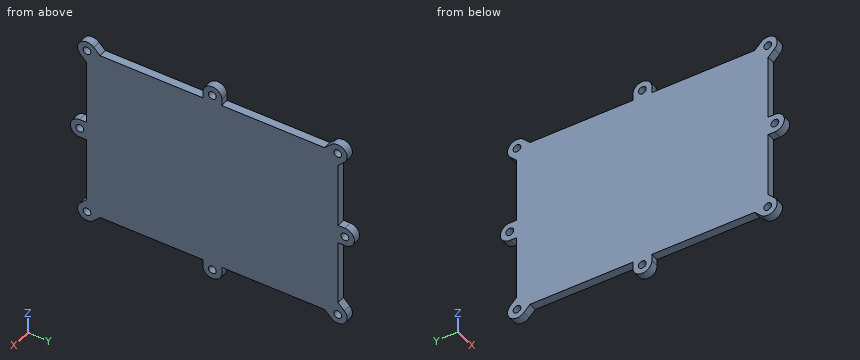
from build123d import *

# Parameters (mm, degrees)
BOSS_EXTRUDE1_DEPTH  = 4.7625
M4_CLEARANCE_HOLE1_D = 4.5


with BuildPart() as part:
    # Sketch1 → Boss-Extrude1 (new body)
    with BuildSketch(Plane(origin=(0, 0, 0), x_dir=(0, 0, -1), z_dir=(1, 0, 0))):
        with BuildLine():
            Line((-12.938571051, 72.8815), (-50.697896458, 72.8815))
            Line((-50.697896458, 72.8815), (-50.697896458, 76.7912))
            ThreePointArc((-50.697896458, 76.7912), (-56.197896458, 82.2912), (-61.697896458, 76.7912))
            Line((-61.697896458, 76.7912), (-61.697896458, 72.8815))
            Line((-61.697896458, 72.8815), (-99.457221865, 72.8815))
            Line((-99.457221865, 72.8815), (-103.084126021, 76.508404156))
            ThreePointArc((-103.084126021, 76.508404156), (-110.862300614, 76.508404156), (-110.862300614, 68.730229563))
            Line((-110.862300614, 68.730229563), (-107.235396458, 65.103325407))
            Line((-107.235396458, 65.103325407), (-107.235396458, 5.5))
            Line((-107.235396458, 5.5), (-111.145096458, 5.5))
            ThreePointArc((-111.145096458, 5.5), (-116.645096458, 0), (-111.145096458, -5.5))
            Line((-111.145096458, -5.5), (-107.235396458, -5.5))
            Line((-107.235396458, -5.5), (-107.235396458, -65.103325407))
            Line((-107.235396458, -65.103325407), (-110.862300614, -68.730229563))
            ThreePointArc((-110.862300614, -68.730229563), (-110.862300614, -76.508404156), (-103.084126021, -76.508404156))
            Line((-103.084126021, -76.508404156), (-99.457221865, -72.8815))
            Line((-99.457221865, -72.8815), (-61.697896458, -72.8815))
            Line((-61.697896458, -72.8815), (-61.697896458, -76.7912))
            ThreePointArc((-61.697896458, -76.7912), (-56.197896458, -82.2912), (-50.697896458, -76.7912))
            Line((-50.697896458, -76.7912), (-50.697896458, -72.8815))
            Line((-50.697896458, -72.8815), (-12.938571051, -72.8815))
            Line((-12.938571051, -72.8815), (-9.311666896, -76.508404156))
            ThreePointArc((-9.311666896, -76.508404156), (-1.533492302, -76.508404156), (-1.533492302, -68.730229563))
            Line((-1.533492302, -68.730229563), (-5.160396458, -65.103325407))
            Line((-5.160396458, -65.103325407), (-5.160396458, -5.5))
            Line((-5.160396458, -5.5), (-1.250696458, -5.5))
            ThreePointArc((-1.250696458, -5.5), (4.249303542, 0), (-1.250696458, 5.5))
            Line((-1.250696458, 5.5), (-5.160396458, 5.5))
            Line((-5.160396458, 5.5), (-5.160396458, 65.103325407))
            Line((-5.160396458, 65.103325407), (-1.533492302, 68.730229563))
            ThreePointArc((-1.533492302, 68.730229563), (-1.533492302, 76.508404156), (-9.311666896, 76.508404156))
            Line((-9.311666896, 76.508404156), (-12.938571051, 72.8815))
        make_face()
    extrude(amount=-BOSS_EXTRUDE1_DEPTH)

    # M4 Clearance Hole1 (through all)
    with Locations(Plane.ZY.offset(4.7625)):
        with Locations((5.422579599, -72.619316859), (1.250696458, 0), (5.422579599, 72.619316859), (106.973213317, 72.619316859), (111.145096458, 0), (106.973213317, -72.619316859), (56.197896458, -76.7912), (56.197896458, 76.7912)):
            Hole(M4_CLEARANCE_HOLE1_D / 2)


solid = part.part
Geometry: final body of the model. Coordinates: model frame, mm. Give positions to 0.01 mm unless a question says otherwise; leave off trailing zeros. Loops run counter-clockwise (first coordinate to the right, second up) from the corner with the lowest first, then second, coordinate; pieces in that order, holes last. Notation, with made-up numbers: M -23,6.5 L 5,6.5 A10 cw 5,21.5 Z; hole C 18,-24.75 d1. An arc over 180 degrees is marked long. Put each result on its own line as item: value.
1) Cut plane A-A, the plane y = 0. Return the cut outline in (x, z), plus the area to 3 significant figures.
Computed values:
outline: M -4.76,-4.25 L 0,-4.25 L 0,-1 L -4.76,-1 Z; M -4.76,3.5 L 0,3.5 L 0,108.9 L -4.76,108.9 Z; M -4.76,113.4 L 0,113.4 L 0,116.65 L -4.76,116.65 Z
area: 533 mm^2
2) Cut plane C-C, the plane z = 43.5. Return the cut outline in (x, y).
Computed values:
outline: M -4.76,-72.88 L 0,-72.88 L 0,72.88 L -4.76,72.88 Z
3) Material intervals for L1, parallel to Y at x = -0.2, z = 107.5; L2, parallel to Z at x = -0.55, y = 75; L3, parallel to Z at x = -1.55, y = -1.5, sorted ascending. Write a range as from..to.
Computed values:
L1: y = -78.09..-74.81, -70.43..-65.37, -5.5..5.5, 65.37..70.43, 74.81..78.09
L2: z = 0.46..10.82, 50.7..54.84, 57.56..61.7, 101.58..111.93
L3: z = -4.04..-0.43, 2.93..109.47, 112.82..116.44
4) First-contact query: P1, Ø2.5, axis at x = -3.5, z = 39, coming from the +Y side; P2, Ø7, axis at y = 72.62, z = 5.42, coming from the +X side; P3, Ø1.2, axis at x = -2, y = -74.5, coming from the +Z side; P4, Ø1.2, axis at x = -2, y = 75.5, coming from the +Z side. Flat tips, straight axial feed; report the tip coordinate or a pass-through.
Computed values:
P1: stops at y = 72.88
P2: stops at x = 0
P3: stops at z = 112.32
P4: stops at z = 111.98
5) Cut plane B-B, the plane y = -24. Return the cut outline in (x, z), plus the area to 3 significant figures.
Computed values:
outline: M -4.76,5.16 L 0,5.16 L 0,107.24 L -4.76,107.24 Z
area: 486 mm^2
